```python
from build123d import *

# Parameters (mm, degrees)
BOSS_EXTRUDE1_DEPTH = 6
FILLET1_R           = 9
SKETCH2_R           = 1.7
CUT_EXTRUDE1_DEPTH  = 178.890415706
SKETCH3_R           = 1.7
CUT_EXTRUDE2_DEPTH  = 178.890415706


with BuildPart() as part:
    # Sketch1 → Boss-Extrude1 (new body)
    with BuildSketch(Plane.XY):
        Polygon((0, 0), (0, 17.5), (-6, 17.5), (-6, 27.5), (0, 27.5), (0, 45), (166, 45), (166, 27.5), (172, 27.5), (172, 17.5), (166, 17.5), (166, 0), (146, 0), (146, 30), (88, 30), (88, 0), (78, 0), (78, 30), (20, 30), (20, 0), align=None)
    extrude(amount=BOSS_EXTRUDE1_DEPTH)

    # Fillet1
    fillet1_edges = [part.edges().sort_by_distance(p)[0] for p in [
        (146, 30, 3),
        (88, 30, 3),
        (78, 30, 3),
        (20, 30, 3),
    ]]
    fillet(fillet1_edges, radius=FILLET1_R)

    # Sketch2 → Cut-Extrude1 (cut, through all)
    with BuildSketch(Plane.XY.offset(6)):
        with Locations((10, 14)):
            Circle(SKETCH2_R)
        with Locations((83, 14)):
            Circle(SKETCH2_R)
        with Locations((156, 14)):
            Circle(SKETCH2_R)
    extrude(amount=-CUT_EXTRUDE1_DEPTH, mode=Mode.SUBTRACT)

    # Sketch3 → Cut-Extrude2 (cut, through all)
    with BuildSketch(Plane.XY.offset(6)):
        with Locations((9, 27)):
            Circle(SKETCH3_R)
    extrude(amount=-CUT_EXTRUDE2_DEPTH, mode=Mode.SUBTRACT)


solid = part.part
```
Part model, mm, in its own coordinate system. A direction names the side the tool comes from. Round coordinates to 2 decimals unless told otherwise and drop trailing zeros. Loops run counter-clockwise (first coordinate to the right, second up) from the corner with the lowest first, then second, coordinate; pieces in that order, holes last. Notation, with made-up numbers: (-8, 83) -> (15, 83) arc R16 ccw to (15, 113) -> close; hole circle Ø1 at (18.25, 72.25). An arc over 180 degrees is marked (long way). Use one line per item in the form item = value. Start each with the question number.
Item 1: Two-plate mould, pull along X, no slides. Class faces 5 (the flat face through (10, 0, 3)), 6 (the flat face through (146, 10, 3)), 7 (the flat face through (172, 23, 3)): released by +X, released by -X, zero draft, split by the parting line, or undercut.
Item 2: Band-saw the part on A-A (y = 9.5). List the corners of the cut face in (x, z), plus the area to 3 significant figures.
Item 3: Band-saw the part on C-C (x = 156). List the corners of the cut face in (y, z), plus the area to 3 significant figures.
Item 4: Band-saw the part on B-B (z = 5). List the corners of the cut face in (x, y), plus the area to 3 significant figures.
Item 5: Band-saw the part on D-D (y = 37.5). List the corners of the cut face in (x, z), plus the area to 3 significant figures.
Item 6: Drill centre lines: line 1 along X through (y, z) = (10, 1.55); line 2 along Y through (x, z) = (156, 4.8); line 3 along Y through (x, z) = (10, 2.4). Where is each one in solid material? Low to high.
Item 7: Drop flat-ended pins along their axis: pin 1 Ø2.5 at (x, y) = (83, 14) entering from +Z; pin 2 Ø3 at (y, z) = (15, 2.5) entering from -X; pin 3 Ø1.5 at (x, y) = (54, 30) entering from -Z; pin 4 Ø1.8 at (x, z) = (111, 1.5) entering from -Y. Give the stop position or say it passes through.
Item 8: Tool access for faces 1 (the cylindrical face through (90.706, 27.434, 3.042)), 2 (the flat face through (0, 36, 3)), 3 (the flat face through (169, 27.5, 3)), 4 (the flat face through (0, 9, 3)): list every direction of +Z, -Z, +X, -X, +Y, -Y with a clear straight run to the whole face (end or side of a thin tool).
Data:
q1.face_5 = zero draft
q1.face_6 = undercut
q1.face_7 = released by +X
q2.outline = (0, 0) -> (20, 0) -> (20, 6) -> (0, 6) -> close; (78, 0) -> (88, 0) -> (88, 6) -> (78, 6) -> close; (146, 0) -> (166, 0) -> (166, 6) -> (146, 6) -> close
q2.area = 300 mm^2
q3.outline = (0, 0) -> (12.3, 0) -> (12.3, 6) -> (0, 6) -> close; (15.7, 0) -> (45, 0) -> (45, 6) -> (15.7, 6) -> close
q3.area = 250 mm^2
q4.outline = (-6, 17.5) -> (0, 17.5) -> (0, 0) -> (20, 0) -> (20, 21) arc R9 cw to (29, 30) -> (69, 30) arc R9 cw to (78, 21) -> (78, 0) -> (88, 0) -> (88, 21) arc R9 cw to (97, 30) -> (137, 30) arc R9 cw to (146, 21) -> (146, 0) -> (166, 0) -> (166, 17.5) -> (172, 17.5) -> (172, 27.5) -> (166, 27.5) -> (166, 45) -> (0, 45) -> (0, 27.5) -> (-6, 27.5) -> close; hole circle Ø3.4 at (9, 27); hole circle Ø3.4 at (10, 14); hole circle Ø3.4 at (83, 14); hole circle Ø3.4 at (156, 14)
q4.area = 4,140 mm^2
q5.outline = (0, 0) -> (166, 0) -> (166, 6) -> (0, 6) -> close
q5.area = 996 mm^2
q6.line_1 = 0 to 20, 78 to 88, 146 to 166
q6.line_2 = 0 to 12.3, 15.7 to 45
q6.line_3 = 0 to 12.3, 15.7 to 25.63, 28.37 to 45
q7.pin_1 = through
q7.pin_2 = 0
q7.pin_3 = 0
q7.pin_4 = 30
q8.face_1 = +Z, -Z, -Y
q8.face_2 = +Z, -Z, -X, +Y
q8.face_3 = +Z, -Z, +X, +Y
q8.face_4 = +Z, -Z, -X, -Y
